```python
from build123d import *

# Parameters (mm, degrees)
BOSS_EXTRU_1_DEPTH      = 4
ESQUISSE2_R             = 10
ENL_V_MAT_EXTRU_1_DEPTH = 227.525936705
ESQUISSE3_R             = 10
ENL_V_MAT_EXTRU_2_DEPTH = 227.525936705


with BuildPart() as part:
    # Esquisse1 → Boss.-Extru.1 (new, symmetric)
    with BuildSketch(Plane.XY):
        with BuildLine():
            Line((-200, 25), (200, 25))
            ThreePointArc((200, 25), (225, 0), (200, -25))
            Line((200, -25), (-200, -25))
            ThreePointArc((-200, -25), (-225, 0), (-200, 25))
        make_face()
    extrude(amount=BOSS_EXTRU_1_DEPTH, both=True)

    # Esquisse2 → Enlèv. mat.-Extru.1 (cut, through all)
    with BuildSketch(Plane.XY.offset(4)):
        with Locations((-200, 0)):
            Circle(ESQUISSE2_R)
        with Locations((200, 0)):
            Circle(ESQUISSE2_R)
    extrude(amount=-ENL_V_MAT_EXTRU_1_DEPTH, mode=Mode.SUBTRACT)

    # Esquisse3 → Enlèv. mat.-Extru.2 (cut, through all)
    with BuildSketch(Plane(origin=(0, 0, -4), x_dir=(-1, 0, 0), z_dir=(0, 0, -1))):
        with Locations((-70, 0)):
            Circle(ESQUISSE3_R)
    extrude(amount=-ENL_V_MAT_EXTRU_2_DEPTH, mode=Mode.SUBTRACT)


solid = part.part
```
Input: part model. Units: mm. Frame: model coordinates. Coordinates: 2 decimals unless noted, no trailing zeros. Write each loop counter-clockwise with the first axis right and the second up, starting at its lowest first coordinate (ties: lowest second). Pieces come first, ordered by that corner, then holes.
1) Material intervals for line 1 along X through (y, z) = (9, -3); line 2 along X through (y, z) = (-8, -2.5); line 3 along Y through (x, z) = (70, 0), sorted ascending.
2) Section A-A on y = 0. Output: boundary loops of the cut face in (x, z), and give its area (3 significant figures).
3) Mould query, pull axis X, two halves, no side actions, for faces 1 (the cylindrical face through (224.994, 0.55, 0.056)), 2 (the flat face through (3, 0, 4)), 3 (the cylindrical face through (-190.763, -3.83, 0.056)). Classes: pulls with the +X half, pulls with the -X half, needs draft (parallel to the pull), parting line crosses it, or undercut.
4) Pin query (flat end, axial travel): pin 1 Ø16 at (x, y) = (200, 0) entering from +Z. Return the tip coordinate at first contact, or that it passes through.
5) Section C-C on z = -2.5. Output: boundary loops of the cut face in (x, y).
6) Section B-B on x = 70. Output: boundary loops of the cut face in (y, z), and give its area (3 significant figures).
Check result:
1. line 1: x = -223.32 to -204.36, -195.64 to 65.64, 74.36 to 195.64, 204.36 to 223.32
1. line 2: x = -223.69 to -206, -194 to 64, 76 to 194, 206 to 223.69
1. line 3: y = -25 to -10, 10 to 25
2. outline: (-225, -4) - (-210, -4) - (-210, 4) - (-225, 4) - close; (-190, -4) - (60, -4) - (60, 4) - (-190, 4) - close; (80, -4) - (190, -4) - (190, 4) - (80, 4) - close; (210, -4) - (225, -4) - (225, 4) - (210, 4) - close
2. area: 3,120 mm2
3. face 1: pulls with the +X half
3. face 2: needs draft
3. face 3: undercut
4. pin 1: passes through
5. outline: (-200, -25) - (200, -25) arc R25 ccw to (200, 25) - (-200, 25) arc R25 ccw to start; hole circle Ø20 at (-200, 0); hole circle Ø20 at (70, 0); hole circle Ø20 at (200, 0)
6. outline: (-25, -4) - (-10, -4) - (-10, 4) - (-25, 4) - close; (10, -4) - (25, -4) - (25, 4) - (10, 4) - close
6. area: 240 mm2
